```python
from build123d import *

# Parameters (mm, degrees)
SKETCH2_R                 = 0.5
CUT_EXTRUDE2_DEPTH        = 21.603397778
F_2_0MM_DOWEL_HOLE1_D     = 2
F_2_0MM_DOWEL_HOLE1_DEPTH = 2
F_2_0MM_DOWEL_HOLE1_TIP   = 0.600860619
CUT_EXTRUDE3_DEPTH        = 21.603397778
CUT_EXTRUDE4_DEPTH        = 10


with BuildPart() as part:
    # Sketch1 → Revolve2 (revolve)
    with BuildSketch(Plane.XY, mode=Mode.PRIVATE) as revolve2_sk:
        with BuildLine():
            Line((0, 0), (-3.5, 0))
            Line((-3.5, 0), (-3.5, 3))
            Line((-3.5, 3), (-1.5, 3))
            Line((-1.5, 3), (-1.5, 3.833209081))
            Line((-1.5, 3.833209081), (-2, 3.833209081))
            Line((-2, 3.833209081), (-2, 7))
            Line((-2, 7), (-1.5, 7))
            Line((-1.5, 7), (-1.5, 19.5))
            ThreePointArc((-1.5, 19.5), (-1.353553391, 19.853553391), (-1, 20))
            Line((-1, 20), (0, 20))
            Line((0, 20), (0, 0))
        make_face()
    revolve(revolve2_sk.sketch.rotate(Axis((0, 7, 0), (0, 1, 0)), 270), axis=Axis((0, 7, 0), (0, 1, 0)))

    # Sketch2 → Cut-Extrude2 (cut, through all)
    with BuildSketch(Plane(origin=(0, 20, 0), x_dir=(1, 0, 0), z_dir=(0, 1, 0))):
        with Locations(Location((0, 0, 0), (0, 0, 270))):
            Circle(SKETCH2_R)
    extrude(amount=-CUT_EXTRUDE2_DEPTH, mode=Mode.SUBTRACT)

    # Ø2.0mm Dowel Hole1
    with Locations(Plane(origin=(0, 0, 0), x_dir=(-1, 0, 0), z_dir=(0, -1, 0))):
        with Locations((0, 0)):
            Hole(F_2_0MM_DOWEL_HOLE1_D / 2, depth=F_2_0MM_DOWEL_HOLE1_DEPTH)
            with Locations((0, 0, -(F_2_0MM_DOWEL_HOLE1_DEPTH + F_2_0MM_DOWEL_HOLE1_TIP / 2))):  # 118° drill point
                Cone(0, F_2_0MM_DOWEL_HOLE1_D / 2, F_2_0MM_DOWEL_HOLE1_TIP, mode=Mode.SUBTRACT)

    # Sketch6 → Cut-Extrude3 (cut, through all)
    with BuildSketch(Plane(origin=(0, 20, 0), x_dir=(1, 0, 0), z_dir=(0, 1, 0))):
        with BuildLine():
            Line((1.802775638, -3), (-1.802775638, -3))
            ThreePointArc((-1.802775638, -3), (0, -3.5), (1.802775638, -3))
        make_face()
        with BuildLine():
            Line((-1.861759264, 2.963756475), (1.802775638, 3))
            ThreePointArc((1.802775638, 3), (-0.034614525, 3.499828829), (-1.861759264, 2.963756475))
        make_face()
    extrude(amount=-CUT_EXTRUDE3_DEPTH, mode=Mode.SUBTRACT)

    # Sketch7 → Cut-Extrude4 (cut)
    with BuildSketch(Plane.XY.offset(3)):
        with BuildLine():
            Line((-6.314985728, 2.627394042), (-6.005388139, 3.404344388))
            Line((-6.005388139, 3.404344388), (-1.5, 3.41660454))
            Line((-1.5, 3.41660454), (-1.5, 2.979046191))
            ThreePointArc((-1.5, 2.979046191), (-3.9114467, 2.857357895), (-6.314985728, 2.627394042))
        make_face()
        with BuildLine():
            Line((5.565529025, 2.710812451), (5.565529025, 3.41660454))
            Line((5.565529025, 3.41660454), (1.5, 3.41660454))
            Line((1.5, 3.41660454), (1.5, 2.979046191))
            ThreePointArc((1.5, 2.979046191), (3.535309383, 2.883501076), (5.565529025, 2.710812451))
        make_face()
    extrude(amount=-CUT_EXTRUDE4_DEPTH, mode=Mode.SUBTRACT)


solid = part.part
```
Can you work these out from the model? Positions are in its coordinate system, mm. A direction names the side the tool comes from. Round coordinates to 2 decimals unless told otherwise and drop trailing zeros. Loops run counter-clockwise (first coordinate to the right, second up) from the corner with the lowest first, then second, coordinate; pieces in that order, holes last. Notation, with made-up numbers: (46.5, 61) -> (62.5, 61) arc R26 cw to (62.5, 100) -> close; hole circle Ø5 at (-32.5, 53.5). An arc over 180 degrees is marked (long way). One line per item, written item: value. Start each with the question number.
1. If we mould it in two halves opening along Y, with no side actions, what happens to faces 4 (the cylindrical face through (-0.45, 13.34, -1.43)), 5 (the cylindrical face through (-0.45, 3.42, -1.43)), 6 (the flat face through (-1, 0, 1)), 7 (the flat face through (0, 3, -2))? For each: pulls with the +Y half, pulls with the -Y half, needs draft (parallel to the pull), parting line crosses it, or undercut.
2. If we section it at B-B, the plane y = 5.5: Write out the boundary of the cut face in (x, z).
3. If we section it at A-A, the plane x = 0: Write out the boundary of the cut face in (y, z), then the cut area to 3 significant figures.
4. If I drill on probe 1 along Y at (x, z) = (0.5, -2.25); probe 2 along X at (y, z) = (14.5, 0); probe 3 along Z at (x, y) = (-1.75, 1), over which ranges is the centre line in solid material (lowest first)?
5. For pin 1 (2 mm diameter, centred on x = 1, z = 2, fed in from +Y); pin 2 (1.5 mm diameter, centred on x = -1, y = 8.5, fed in from -Z); pin 3 (1.5 mm diameter, centred on x = -2, y = 5, fed in from -Z), each with a flat end and sliding along its axis, tell me the tip position at first contact or that it passes through.
6. For faces 1 (the flat face through (0, 2, 3)), 2 (the cylindrical face through (2, 5, 0)), 3 (the cylindrical face through (0, 1, 1)), which set-ups out of +Z, -Z, +X, -X, +Y, -Y let a thin tool reach every point of the face, with its end or its side?
7. If we section it at D-D, the plane x = 2.5: Write out the boundary of the cut face in (y, z), then the cut area to 3 significant figures.
8. If we section it at C-C, the plane y = 17.75: Write out the boundary of the cut face in (x, z).
Calculated:
1. face 4: needs draft
1. face 5: undercut
1. face 6: pulls with the -Y half
1. face 7: undercut
2. outline: circle Ø4 at (0, 0); hole circle Ø1 at (0, 0)
3. outline: (0, -2.98) -> (3, -2.98) -> (3, -1.5) -> (3.83, -1.5) -> (3.83, -2) -> (7, -2) -> (7, -1.5) -> (19.5, -1.5) arc R0.5 ccw to (20, -1) -> (20, -0.5) -> (2.3, -0.5) -> (2, -1) -> (0, -1) -> close; (0, 1) -> (2, 1) -> (2.3, 0.5) -> (20, 0.5) -> (20, 1) arc R0.5 ccw to (19.5, 1.5) -> (7, 1.5) -> (7, 2) -> (3.83, 2) -> (3.83, 1.5) -> (3, 1.5) -> (3, 3) -> (0, 3) -> close
3. area: 49.9 mm²
4. probe 1: y = 0 to 3
4. probe 2: x = -1.5 to -0.5, 0.5 to 1.5
4. probe 3: z = -2.96 to 3
5. pin 1: stops at y = 19.94
5. pin 2: stops at z = -1.48
5. pin 3: stops at z = -1.56
6. face 1: +Z, +X, -X, +Y, -Y
6. face 2: +Y
6. face 3: -Y
7. outline: (0, -2.45) -> (2.94, -2.45) -> (2.94, 2.45) -> (0, 2.45) -> close
7. area: 14.4 mm²
8. outline: circle Ø3 at (0, 0); hole circle Ø1 at (0, 0)
